Part model, mm, in its own coordinate system. Face numbers are marked on the shaded views. Coordinates: 2 decimals unless noted, no trailing zeros. Write each loop counter-clockwise with the first axis right and the second up, starting at its lowest first coordinate (ties: lowest second). Pieces come first, ordered by that corner, then holes. Notation, with made-up numbers: (81.25, 19) -> (87.25, 19) arc R11 ccw to (87.25, 36) -> close; hole circle Ø2 at (2.5, 44). An arc over 180 degrees is marked (long way). Write item = value, one per line.
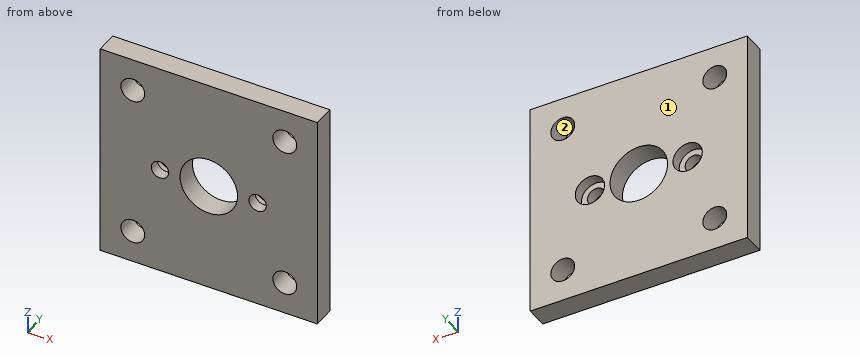
from build123d import *

# Parameters (mm, degrees)
SKETCH_1_W          = 20
SKETCH_1_H          = 20
SKETCH_1_R          = 0.8
SKETCH_1_R_2        = 2.65
EXTRUDE_1_DEPTH     = 2
SKETCH_2_R          = 1.35
CUT_EXTRUDE_1_DEPTH = 1
SKETCH_3_R          = 1.1
CUT_EXTRUDE_2_DEPTH = 15.282856857


with BuildPart() as part:
    # 草图1 → 凸台-拉伸1 (new body)
    with BuildSketch(Plane(origin=(0, 0, 0), x_dir=(1, 0, 0), z_dir=(0, 1, 0))):
        Rectangle(SKETCH_1_W, SKETCH_1_H)
        with Locations(Location((-4.5, 0, 0), (0, 0, 270))):
            Circle(SKETCH_1_R, mode=Mode.SUBTRACT)
        with Locations(Location((4.5, 0, 0), (0, 0, 270))):
            Circle(SKETCH_1_R, mode=Mode.SUBTRACT)
        with Locations(Location((0, 0, 0), (0, 0, 270))):
            Circle(SKETCH_1_R_2, mode=Mode.SUBTRACT)
    extrude(amount=EXTRUDE_1_DEPTH)

    # 草图2 → 切除-拉伸1 (cut)
    with BuildSketch(Plane(origin=(0, 2, 0), x_dir=(1, 0, 0), z_dir=(0, 1, 0))):
        with Locations(Location((-4.5, 0, 0), (0, 0, 270))):
            Circle(SKETCH_2_R)
        with Locations(Location((4.5, 0, 0), (0, 0, 270))):
            Circle(SKETCH_2_R)
    extrude(amount=-CUT_EXTRUDE_1_DEPTH, mode=Mode.SUBTRACT)

    # 草图3 → 切除-拉伸2 (cut, through all)
    with BuildSketch(Plane.XZ):
        with Locations(Location((-7, 7, 0), (0, 0, 270))):
            Circle(SKETCH_3_R)
        with Locations(Location((7, 7, 0), (0, 0, 270))):
            Circle(SKETCH_3_R)
        with Locations(Location((7, -7, 0), (0, 0, 270))):
            Circle(SKETCH_3_R)
        with Locations(Location((-7, -7, 0), (0, 0, 270))):
            Circle(SKETCH_3_R)
    extrude(amount=-CUT_EXTRUDE_2_DEPTH, mode=Mode.SUBTRACT)


solid = part.part
Q1. Saw through at C-C on z = -7. Give the cut face in (x, y), and give its area (3 significant figures).
Model answer:
outline = (-10, 0) -> (-8.1, 0) -> (-8.1, 2) -> (-10, 2) -> close; (-5.9, 0) -> (5.9, 0) -> (5.9, 2) -> (-5.9, 2) -> close; (8.1, 0) -> (10, 0) -> (10, 2) -> (8.1, 2) -> close
area = 31.2 mm²
Q2. Saw through at D-D on y = 0.35. Give the cut face in (x, z), and give its area (3 significant figures).
Model answer:
outline = (-10, -10) -> (10, -10) -> (10, 10) -> (-10, 10) -> close; hole circle Ø2.2 at (-7, -7); hole circle Ø2.2 at (-7, 7); hole circle Ø1.6 at (-4.5, 0); hole circle Ø5.3 at (0, 0); hole circle Ø1.6 at (4.5, 0); hole circle Ø2.2 at (7, -7); hole circle Ø2.2 at (7, 7)
area = 359 mm²
Q3. Mould opens along Z. For the marked faces 1 and 2 say: released by +Z, released by -Z, zero draft, split by the parting line, or undercut.
Model answer:
face_1 = zero draft
face_2 = undercut
Q4. Saw through at B-B on x = 4.5. Give the cut face in (y, z).
Model answer:
outline = (0, -10) -> (2, -10) -> (2, -1.35) -> (1, -1.35) -> (1, -0.8) -> (0, -0.8) -> close; (0, 0.8) -> (1, 0.8) -> (1, 1.35) -> (2, 1.35) -> (2, 10) -> (0, 10) -> close
Q5. Saw through at A-A on z = 0. Give the cut face in (x, y).
Model answer:
outline = (-10, 0) -> (-5.3, 0) -> (-5.3, 1) -> (-5.85, 1) -> (-5.85, 2) -> (-10, 2) -> close; (-3.7, 0) -> (-2.65, 0) -> (-2.65, 2) -> (-3.15, 2) -> (-3.15, 1) -> (-3.7, 1) -> close; (2.65, 0) -> (3.7, 0) -> (3.7, 1) -> (3.15, 1) -> (3.15, 2) -> (2.65, 2) -> close; (5.3, 0) -> (10, 0) -> (10, 2) -> (5.85, 2) -> (5.85, 1) -> (5.3, 1) -> close
Q6. Probe line 1 (X direction, y = 1.25, z = -7); line 2 (Z direction, x = 4.5, y = 0.65); line 3 (Z direction, x = -8, y = 1.95). List the from-to ranges inside material, lowest first. Write a range as from..to.
Model answer:
line_1 = -10..-8.1, -5.9..5.9, 8.1..10
line_2 = -10..-0.8, 0.8..10
line_3 = -10..-7.46, -6.54..6.54, 7.46..10
Q7. Pin check, flat tip, straight feed: pin 1 (1.8 mm diameter, centred on x = 4.5, z = 0, fed in from +Y). Stop position of the tip, or through.
Model answer:
pin_1 = 1
